Build history of the part. All positions in model axes, mm. Face numbers are marked on the shaded views. A direction names the side the tool comes from. Give positions to 0.01 mm unless a question says otherwise; leave off trailing zeros. Order: outer loops, then holes, each group sorted by start corner. A loop starts at its lowest first (then second) coordinate and runs counter-clockwise, first axis right, second up. Notation, with made-up numbers: (75.5, 18) - (86.5, 18) arc R28 cw to (86.5, 39) - close; hole circle Ø11 at (-7, 81). An arc over 180 degrees is marked (long way). Answer in a Markdown table with one row per item.
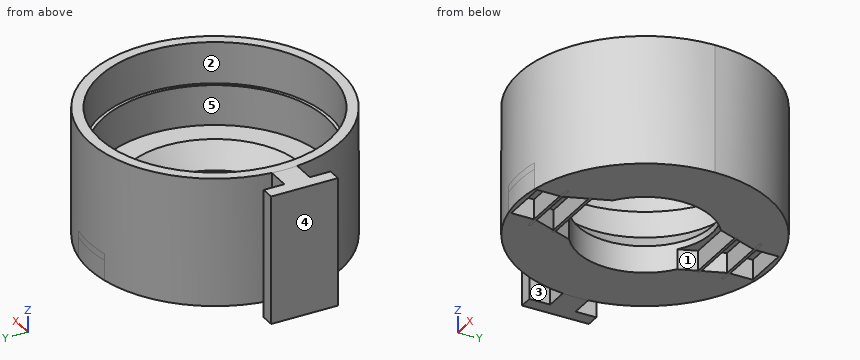
```python
from build123d import *

# Parameters (mm, degrees)
F0_R      = 11.938
F1_DEPTH  = 12.192
F2_R      = 6.35
F3_DEPTH  = 12.193
F4_R      = 10.6045
F5_DEPTH  = 7.747
F6_SIZE   = 1.905
F7_R      = 10.922
F8_DEPTH  = 3.937
F9_W      = 4.445
F9_H      = 23.876
F10_DEPTH = 1.905
F13_DEPTH = 1.905
F14_W     = 6.604
F14_H     = 0.254
F15_DEPTH = 2.54
F17_DEPTH = 12.192


with BuildPart() as f1:
    # F0 (on Top) → F1 (new body)
    with BuildSketch(Plane.XY):
        Circle(F0_R)
    extrude(amount=-F1_DEPTH)

    # F2 (on face) → F3 (cut, through all)
    with BuildSketch(Plane.XY):
        Circle(F2_R)
    extrude(amount=-F3_DEPTH, mode=Mode.SUBTRACT)

    # F4 (on face) → F5 (cut)
    with BuildSketch(Plane.XY):
        Circle(F4_R)
    extrude(amount=-F5_DEPTH, mode=Mode.SUBTRACT)

    # F6
    f6_edges = [f1.edges().sort_by_distance(p)[0] for p in [
        (-6.35, 0, -7.747),
    ]]
    chamfer(f6_edges, length=F6_SIZE)

    # F7 (on Top) → F8 (cut)
    with BuildSketch(Plane.XY):
        Circle(F7_R)
    extrude(amount=-F8_DEPTH, mode=Mode.SUBTRACT)

    # F9 (on face) → F10 (cut)
    with BuildSketch(Plane(origin=(0, 0, -12.192), x_dir=(1, 0, 0), z_dir=(0, 0, -1))):
        Rectangle(F9_W, F9_H)
    extrude(amount=-F10_DEPTH, mode=Mode.SUBTRACT)

    # F12 (on offset) → F13 (cut)
    with BuildSketch(Plane(origin=(0, 0, -12.192), x_dir=(1, 0, 0), z_dir=(0, 0, -1))):
        Polygon((0, 9.144), (-2.2225, 9.144), (-5.08, 1.524), (0, 1.524), align=None)
        Polygon((2.2225, 9.144), (0, 9.144), (0, 1.524), (5.08, 1.524), align=None)
        Polygon((0, -9.144), (2.2225, -9.144), (5.08, -1.524), (0, -1.524), (-5.08, -1.524), (-2.2225, -9.144), align=None)
    extrude(amount=-F13_DEPTH, mode=Mode.SUBTRACT)

    # F14 (on offset) → F15 (join)
    with BuildSketch(Plane(origin=(0, 0, -12.192), x_dir=(1, 0, 0), z_dir=(0, 0, -1))):
        with BuildLine():
            ThreePointArc((2.2225, 11.7292940005), (0, 11.938), (-2.2225, 11.7292940005))
            Line((-2.2225, 11.7292940005), (-2.2225, 11.4752940005))
            Line((-2.2225, 11.4752940005), (2.2225, 11.4752940005))
            Line((2.2225, 11.4752940005), (2.2225, 11.7292940005))
        make_face()
        with Locations((0, 9.1892940005)):
            Rectangle(F14_W, F14_H)
        with Locations((0, 6.9032940005)):
            Rectangle(F14_W, F14_H)
        with Locations((0, -6.9032940005)):
            Rectangle(F14_W, F14_H)
        with Locations((0, -9.1892940005)):
            Rectangle(F14_W, F14_H)
        with BuildLine():
            ThreePointArc((-2.2225, -11.7292940005), (0, -11.938), (2.2225, -11.7292940005))
            Line((2.2225, -11.7292940005), (2.2225, -11.4752940005))
            Line((2.2225, -11.4752940005), (-2.2225, -11.4752940005))
            Line((-2.2225, -11.4752940005), (-2.2225, -11.7292940005))
        make_face()
    extrude(amount=-F15_DEPTH)

    # F16 (on Top) → F17 (join)
    with BuildSketch(Plane.XY):
        with BuildLine():
            ThreePointArc((-11.8768767675, -1.2065), (-11.938, 0), (-11.8768767675, 1.2065))
            Line((-11.8768767675, 1.2065), (-14.0358767675, 1.2065))
            Line((-14.0358767675, 1.2065), (-14.0358767675, 3.175))
            Line((-14.0358767675, 3.175), (-15.3058767675, 3.175))
            Line((-15.3058767675, 3.175), (-15.3058767675, 0))
            Line((-15.3058767675, 0), (-15.3058767675, -3.175))
            Line((-15.3058767675, -3.175), (-14.0358767675, -3.175))
            Line((-14.0358767675, -3.175), (-14.0358767675, -1.2065))
            Line((-14.0358767675, -1.2065), (-11.8768767675, -1.2065))
        make_face()
    extrude(amount=-F17_DEPTH)


solid = f1.part
```
1. Two-plate mould, pull along Y, no slides. Class the marked faces 1, 2 and 3: +Y half, -Y half, draft (parallel to the pull), parting line (faces both ways), or undercut.
Check result:
| item | result |
|---|---|
| face 1 | undercut |
| face 2 | undercut |
| face 3 | draft |
2. Which spindle directions (+Z, -Z, +X, -X, +Y, -Y) get a long thin tool onto all of the face, cutting with end or side? Do the marked faces 4 and 5. Say none if no direction does.
Check result:
| item | result |
|---|---|
| face 4 | +Z, -Z, -X, +Y, -Y |
| face 5 | +Z |
3. Drop flat-ended pins along their axis: P1, Ø1.5, axis at y = -10, z = -11, coming from the +X side; P2, Ø1, axis at y = 2, z = -6.5, coming from the +X side; P3, Ø6, axis at x = 1.5, y = 6.5, coming from the +Z side. Give the stop position or say it passes through.
Check result:
| item | result |
|---|---|
| P1 | stops at x = 7.55 |
| P2 | stops at x = 11.84 |
| P3 | stops at z = -7.75 |
4. Cut at B-B on x = -9.75. Write the cut outline in (y, z), and give its area (3 significant figures).
Check result:
| item | result |
|---|---|
| outline | (-6.89, -12.19) - (6.89, -12.19) - (6.89, 0) - (4.92, 0) - (4.92, -3.94) - (4.17, -3.94) - (4.17, -7.75) - (-4.17, -7.75) - (-4.17, -3.94) - (-4.92, -3.94) - (-4.92, 0) - (-6.89, 0) - close |
| area | 97.4 mm² |
5. Cut at D-D on x = 9. Write the cut outline in (y, z).
Check result:
| item | result |
|---|---|
| outline | (-7.84, -12.19) - (7.84, -12.19) - (7.84, 0) - (6.19, 0) - (6.19, -3.94) - (5.61, -3.94) - (5.61, -7.75) - (-5.61, -7.75) - (-5.61, -3.94) - (-6.19, -3.94) - (-6.19, 0) - (-7.84, 0) - close |
6. Cut at C-C on y = -9.75. Write the cut outline in (x, z).
Check result:
| item | result |
|---|---|
| outline | (-6.89, -12.19) - (-2.22, -12.19) - (-2.22, -10.29) - (2.22, -10.29) - (2.22, -12.19) - (6.89, -12.19) - (6.89, 0) - (4.92, 0) - (4.92, -3.94) - (4.17, -3.94) - (4.17, -7.75) - (-4.17, -7.75) - (-4.17, -3.94) - (-4.92, -3.94) - (-4.92, 0) - (-6.89, 0) - close |
7. Cut at A-A on z = -6.5. Write the cut outline in (x, y) (1 decimal), and give its area (3 significant figures).
Check result:
| item | result |
|---|---|
| outline | (-15.3, -3.2) - (-14, -3.2) - (-14, -1.2) - (-11.9, -1.2) arc R11.9 ccw (long way) to (-11.9, 1.2) - (-14, 1.2) - (-14, 3.2) - (-15.3, 3.2) - close; hole circle Ø21.2 at (0, 0) |
| area | 108 mm² |
8. Probe line 1 (Y direction, x = 0, z = -2.35); line 2 (X direction, y = 0, z = -10.9); line 3 (X direction, y = 3, z = -7.25). List the from-to ranges inside material, lowest first.
Check result:
| item | result |
|---|---|
| line 1 | y = -11.94 to -10.92, 10.92 to 11.94 |
| line 2 | x = -15.31 to -6.35, 6.35 to 11.94 |
| line 3 | x = -15.31 to -14.04, -11.55 to -10.17, 10.17 to 11.55 |
